from build123d import *

# Parameters (mm, degrees)
SKETCH001_R   = 30.15
PAD_DEPTH     = 65.85
SKETCH002_R   = 24.15
POCKET_DEPTH  = 53.85
SKETCH003_R   = 30.5
SKETCH003_R_2 = 24.15
PAD001_DEPTH  = 23


with BuildPart() as part:
    # Sketch001 → Pad (new body)
    with BuildSketch(Plane.XY):
        Circle(SKETCH001_R)
    extrude(amount=PAD_DEPTH)

    # Sketch002 (on Face2 of Pad) → Pocket (cut)
    with BuildSketch(Plane(origin=(0, 0, 0), x_dir=(1, 0, 0), z_dir=(0, 0, -1))):
        Circle(SKETCH002_R)
    extrude(amount=-POCKET_DEPTH, mode=Mode.SUBTRACT)

    # Sketch003 → Pad001 (join)
    with BuildSketch(Plane.YZ):
        with Locations((0, 90)):
            Circle(SKETCH003_R)
        with Locations((0, 90)):
            Circle(SKETCH003_R_2, mode=Mode.SUBTRACT)
    extrude(amount=PAD001_DEPTH)


solid = part.part
Geometry: final body of the model. Coordinates: model frame, mm. A direction names the side the tool comes from. Round coordinates to 2 decimals unless told otherwise and drop trailing zeros. Loops run counter-clockwise (first coordinate to the right, second up) from the corner with the lowest first, then second, coordinate; pieces in that order, holes last. Notation, with made-up numbers: M -26.5,29.5 L 11.5,29.5 A17 cw 11.5,35.5 Z; hole C -9,54 d5. An arc over 180 degrees is marked long. One line per question, with ' | ' between items.
(1) Cut plane B-B on y = -25.5. Return the cut outline in (x, z).
Check result:
outline: M -16.09,0 L 16.09,0 L 16.09,65.85 L -16.09,65.85 Z; M 0,73.27 L 23,73.27 L 23,106.73 L 0,106.73 Z
(2) Material intervals for line 1 along Z through (x, y) = (11, 0); line 2 along Y through (x, z) = (0, 28.5); line 3 along Z through (x, y) = (1.5, -25), sorted ascending. Write a range as from..to.
Check result:
line 1: z = 53.85..65.85, 114.15..120.5 | line 2: y = -30.15..-24.15, 24.15..30.15 | line 3: z = 0..65.85, 72.53..107.47
(3) Access query for faces 1 (the flat face through (0, 25, 0)), 2 (the cylindrical face through (-24.127, -1.062, 26.548)), 3 (the flat face through (23, -11, 112)). Directions: +Z, -Z, +X, -X, +Y, -Y. A direction counts if a zero-diameter tool reaches every point of the face in a straight line with its end or side. Return the directions, or none.
Check result:
face 1: -Z, +X, -X, +Y, -Y | face 2: -Z | face 3: +Z, +X, +Y, -Y
(4) Contact query for flat-ended pins moving along their axis: P1, Ø1, axis at y = -12.5, z = 29.5, coming from the -X side; P2, Ø5, axis at x = 1.5, y = 0, coming from the -Z side; P3, Ø12, axis at y = -23.5, z = 63.5, coming from the -X side. Output: stop coordinate, or through.
Check result:
P1: stops at x = -27.66 | P2: stops at z = 53.85 | P3: stops at x = -24.55
(5) Cut plane D-D on z = 36.5. Return the cut outline in (x, y).
Check result:
outline: C 0,0 d60.3; hole C 0,0 d48.3
(6) Cut plane C-C on x = 14.5. Return the cut outline in (y, z).
Check result:
outline: M -26.43,0 L -19.31,0 L -19.31,53.85 L 19.31,53.85 L 19.31,0 L 26.43,0 L 26.43,65.85 L 18.63,65.85 A30.5 ccw long -18.63,65.85 L -26.43,65.85 Z; hole C 0,90 d48.3
(7) Cut plane A-A on z = 90. Return the cut outline in (x, y).
Check result:
outline: M 0,-30.5 L 23,-30.5 L 23,-24.15 L 0,-24.15 Z; M 0,24.15 L 23,24.15 L 23,30.5 L 0,30.5 Z
(8) Pull-direction query (Y, two-part tool) for faces 4 (the cylindrical face through (-6.536, -29.433, 32.464)), 5 (the cylindrical face through (11.339, -5.235, 66.424)), 6 (the flat face through (0, -11, 112)); classes: +Y half, -Y half, draft (parallel to the pull), parting line (faces both ways), or undercut.
Check result:
face 4: parting line | face 5: undercut | face 6: draft
